Design review of the part shown in the three views and the two pictorial views. Dimensions are in mm from the part's minimum x, y and z. Coordinates: 2 decimals unless noted, no trailing zeros. Loops run counter-clockwise (first coordinate to the right, second up) from the corner with the lowest first, then second, coordinate; pieces in that order, holes last. Notation, with made-up numbers: M 56,23 L 93,23 A13 ccw 93,32 Z; hole C 1.25,21.5 d9. An arc over 180 degrees is marked long. Put each result on its own line as item: value. Start each with the question number.
(1) Clearance check with flat-ended pins moving along their axes: pin 1 (10 mm diameter, centred on y = 8.5, z = 14.5, fed in from -X); pin 2 (2 mm diameter, centred on x = 5.5, z = 94.5, fed in from -Y); pin 3 (6 mm diameter, centred on x = 26, y = 15, fed in from +Z); pin 4 (7.5 mm diameter, centred on x = 30.5, z = 90.5, fed in from +Y). State where each tip first meets the part, or that it passes through.
(2) For probe 1 along X at (y, z) = (24, 94.5); probe 2 along Z at (x, y) = (5.5, 20.5); probe 3 along Z at (x, y) = (75.5, 22.75), list the stretches that pass through material, from the lowest coordinate up. Write a range as [from, to].
(3) Take a section at A-A, the plane x = 75.5. Give the boundary of the cut face in (y, z), then the cut area to 4 significant figures.
(4) The part is to be moulded in two halves that separate along X. For the marked faces 1, 2, 3 and 4, say which applies: +X half, -X half, draft (parallel to the pull), parting line (faces both ways), or undercut.
(5) Take a section at B-B, the plane y = 26.5. Give the boundary of the cut face in (x, z).
(6) Take a section at C-C, the plane z = 94.5. Give the boundary of the cut face in (x, y).
(7) Take a section at D-D, the plane x = 50. Give the boundary of the cut face in (y, z).
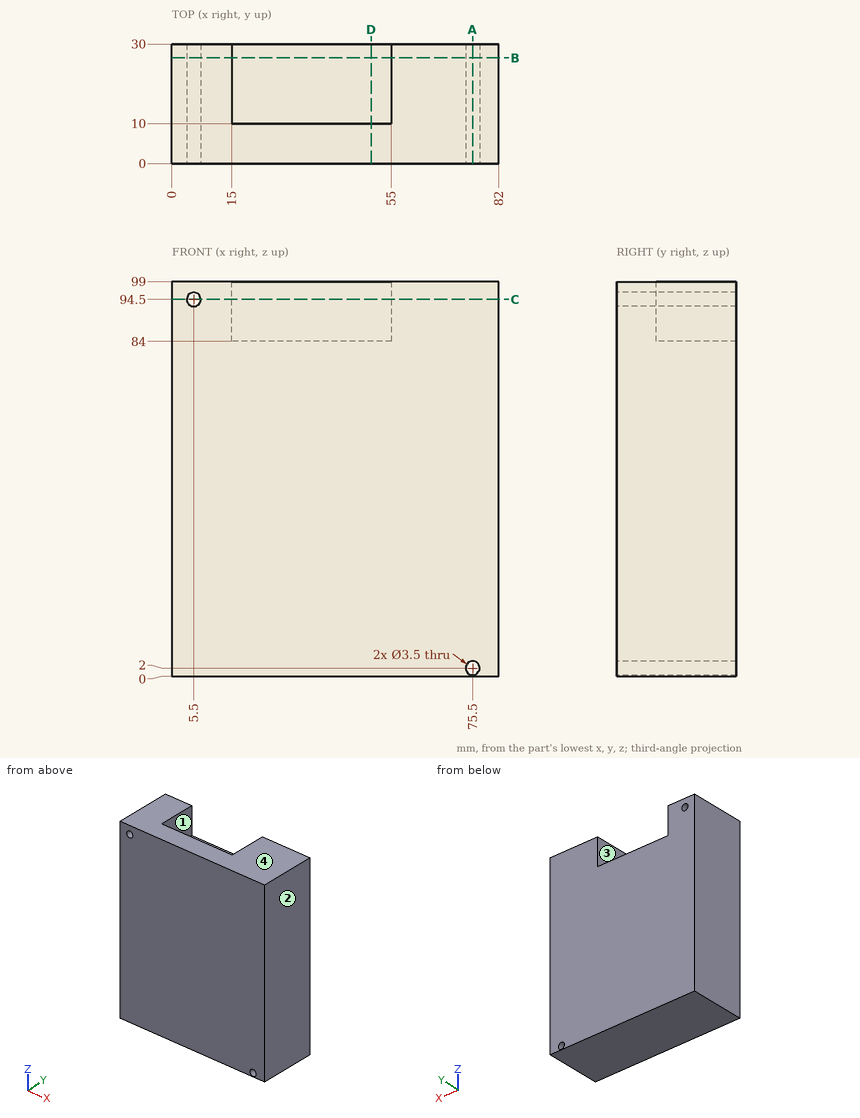
Computed values:
1. pin 1: stops at x = 0
1. pin 2: passes through
1. pin 3: stops at z = 84
1. pin 4: stops at y = 10
2. probe 1: x = [0, 3.75], [7.25, 15], [55, 82]
2. probe 2: z = [0, 92.75], [96.25, 99]
2. probe 3: z = [0, 0.25], [3.75, 99]
3. outline: M 0,0 L 30,0 L 30,0.25 L 0,0.25 Z; M 0,3.75 L 30,3.75 L 30,99 L 0,99 Z
3. area: 2,865 mm^2
4. face 1: undercut
4. face 2: +X half
4. face 3: undercut
4. face 4: draft
5. outline: M 0,0 L 82,0 L 82,99 L 55,99 L 55,84 L 15,84 L 15,99 L 0,99 Z; hole C 5.5,94.5 d3.5; hole C 75.5,2 d3.5
6. outline: M 0,0 L 3.75,0 L 3.75,30 L 0,30 Z; M 7.25,0 L 82,0 L 82,30 L 55,30 L 55,10 L 15,10 L 15,30 L 7.25,30 Z
7. outline: M 0,0 L 30,0 L 30,84 L 10,84 L 10,99 L 0,99 Z
